```python
from build123d import *

# Parameters (mm, degrees)
SKETCH1_R           = 11
SKETCH1_R_2         = 2.5
SKETCH1_R_3         = 1.25
BOSS_EXTRUDE1_DEPTH = 3
CUT_EXTRUDE1_START  = -1
SKETCH2_R           = 11
CUT_EXTRUDE1_DEPTH  = 1


with BuildPart() as part:
    # Sketch1 → Boss-Extrude1 (new body)
    with BuildSketch(Plane(origin=(0, 0, 0), x_dir=(1, 0, 0), z_dir=(0, 1, 0))):
        with Locations(Location((0, 0, 0), (0, 0, 270))):
            Circle(SKETCH1_R)
        with Locations(Location((0, 0, 0), (0, 0, 270))):
            Circle(SKETCH1_R_2, mode=Mode.SUBTRACT)
        with Locations(Location((0, 7, 0), (0, 0, 270))):
            Circle(SKETCH1_R_3, mode=Mode.SUBTRACT)
        with Locations(Location((7, 0, 0), (0, 0, 270))):
            Circle(SKETCH1_R_3, mode=Mode.SUBTRACT)
        with Locations(Location((0, -7, 0), (0, 0, 270))):
            Circle(SKETCH1_R_3, mode=Mode.SUBTRACT)
        with Locations(Location((-7, 0, 0), (0, 0, 270))):
            Circle(SKETCH1_R_3, mode=Mode.SUBTRACT)
    extrude(amount=BOSS_EXTRUDE1_DEPTH)

    # Sketch2 → Cut-Extrude1 (cut)
    with BuildSketch(Plane(origin=(0, 3, 0), x_dir=(1, 0, 0), z_dir=(0, 1, 0)).offset(CUT_EXTRUDE1_START)):
        with Locations(Location((0, 0, 0), (0, 0, 270))):
            Circle(SKETCH2_R)
    extrude(amount=CUT_EXTRUDE1_DEPTH, mode=Mode.SUBTRACT)


solid = part.part
```
Check sheet for the modelled part. Datum: model origin and axes. Units: mm. Round coordinates to 2 decimals unless told otherwise and drop trailing zeros. Loops run counter-clockwise (first coordinate to the right, second up) from the corner with the lowest first, then second, coordinate; pieces in that order, holes last. Notation, with made-up numbers: M -27,-16 L -9,-16 A13 cw -9,8 Z; hole C 77,39.25 d5. An arc over 180 degrees is marked long. Answer as a JSON object with one key per item and string values.
1. Mould release check, pull along X, two halves, no side actions. Record for faces 1 (the cylindrical face through (0.05, 0.99, 5.75)), 2 (the flat face through (3, 0, 0)), 3 (the cylindrical face through (-10.74, 0.99, -2.38)): pulls with the +X half, pulls with the -X half, needs draft (parallel to the pull), parting line crosses it, or undercut.
Reply:
{"face 1": "undercut", "face 2": "needs draft", "face 3": "parting line crosses it"}
2. Scan lines: line 1 (X direction, y = 0.7, z = 0); line 2 (X direction, y = 0.55, z = 8); line 3 (Z direction, x = 1.5, y = 0.5). Record each from-to range of solid material in increasing order.
Reply:
{"line 1": "x = -11 to -8.25, -5.75 to -2.5, 2.5 to 5.75, 8.25 to 11", "line 2": "x = -7.55 to -0.75, 0.75 to 7.55", "line 3": "z = -10.9 to -2, 2 to 10.9"}
3. Section check D-D (y = 1.5). Record the boundary of the cut face in (x, z), plus the area to 3 significant figures.
Reply:
{"outline": "C 0,0 d22; hole C -7,0 d2.5; hole C 0,0 d5; hole C 0,-7 d2.5; hole C 0,7 d2.5; hole C 7,0 d2.5", "area": "341 mm²"}
4. Section check B-B (x = 0). Record the boundary of the cut face in (y, z).
Reply:
{"outline": "M 0,-11 L 2,-11 L 2,-8.25 L 0,-8.25 Z; M 0,-5.75 L 2,-5.75 L 2,-2.5 L 0,-2.5 Z; M 0,2.5 L 2,2.5 L 2,5.75 L 0,5.75 Z; M 0,8.25 L 2,8.25 L 2,11 L 0,11 Z"}
5. Section check A-A (z = 0). Record the boundary of the cut face in (x, y), plus the area to 3 significant figures.
Reply:
{"outline": "M -11,0 L -8.25,0 L -8.25,2 L -11,2 Z; M -5.75,0 L -2.5,0 L -2.5,2 L -5.75,2 Z; M 2.5,0 L 5.75,0 L 5.75,2 L 2.5,2 Z; M 8.25,0 L 11,0 L 11,2 L 8.25,2 Z", "area": "24.0 mm²"}
6. Section check C-C (x = -2.25). Record the boundary of the cut face in (y, z).
Reply:
{"outline": "M 0,-10.77 L 2,-10.77 L 2,-1.09 L 0,-1.09 Z; M 0,1.09 L 2,1.09 L 2,10.77 L 0,10.77 Z"}
